Verification items for the finished model (mm, model axes). Coordinates: 2 decimals unless noted, no trailing zeros. Write each loop counter-clockwise with the first axis right and the second up, starting at its lowest first coordinate (ties: lowest second). Pieces come first, ordered by that corner, then holes. Notation, with made-up numbers: (35, -20) -> (78, -20) arc R25 cw to (78, -8) -> close; hole circle Ø10 at (54, 9.25). An arc over 180 degrees is marked (long way). Answer in a Markdown table with one row per item.
```python
from build123d import *

# Parameters (mm, degrees)
F1_DEPTH = 49


with BuildPart() as f1:
    # F0 (on Top) → F1 (new body)
    with BuildSketch(Plane.XY):
        with BuildLine():
            ThreePointArc((-1.772759, -1.023503), (-0.823705, -3.314722), (-0.5, -5.773503))
            Line((-0.5, -5.773503), (0.5, -5.773503))
            ThreePointArc((0.5, -5.773503), (0.823705, -3.314722), (1.772759, -1.023503))
            ThreePointArc((1.772759, -1.023503), (0, -2.047005), (-1.772759, -1.023503))
        make_face()
        with BuildLine():
            Line((-4.75, 3.319764), (-5.25, 2.453739))
            ThreePointArc((-5.25, 2.453739), (-3.282486, 0.944012), (-1.772759, -1.023503))
            ThreePointArc((-1.772759, -1.023503), (-1.772759, 1.023503), (0, 2.047005))
            ThreePointArc((0, 2.047005), (-2.458781, 2.37071), (-4.75, 3.319764))
        make_face()
        with BuildLine():
            ThreePointArc((0, 2.047005), (-1.772759, 1.023503), (-1.772759, -1.023503))
            ThreePointArc((-1.772759, -1.023503), (0, -2.047005), (1.772759, -1.023503))
            ThreePointArc((1.772759, -1.023503), (1.977255, -0.529804), (2.047005, 0))
            ThreePointArc((2.047005, 0), (1.447451, 1.447451), (0, 2.047005))
        make_face()
        with BuildLine():
            ThreePointArc((4.75, 3.319764), (2.458781, 2.37071), (0, 2.047005))
            ThreePointArc((0, 2.047005), (1.447451, 1.447451), (2.047005, 0))
            ThreePointArc((2.047005, 0), (1.977255, -0.529804), (1.772759, -1.023503))
            ThreePointArc((1.772759, -1.023503), (3.282486, 0.944012), (5.25, 2.453739))
            Line((5.25, 2.453739), (4.75, 3.319764))
        make_face()
    extrude(amount=-F1_DEPTH)


solid = f1.part
```
1. Section check A-A, the plane z = -23. Record the boundary of the cut face in (x, y), plus the area to 3 significant figures.
Geometry says:
| item | result |
|---|---|
| outline | (-5.25, 2.45) arc R9.5 cw to (-1.77, -1.02) arc R9.5 cw to (-0.5, -5.77) -> (0.5, -5.77) arc R9.5 cw to (1.77, -1.02) arc R9.5 cw to (5.25, 2.45) -> (4.75, 3.32) arc R9.5 cw to (0, 2.05) arc R9.5 cw to (-4.75, 3.32) -> close |
| area | 31.4 mm^2 |
2. Section check C-C, the plane y = -1.75. Record the boundary of the cut face in (x, z).
Geometry says:
| item | result |
|---|---|
| outline | (-1.39, -49) -> (1.39, -49) -> (1.39, 0) -> (-1.39, 0) -> close |
3. Thickness scan on line 1 (Y direction, x = 0.25, z = -8); line 2 (X direction, y = 3, z = -24.5). Record the ranges inside material, lowest first. Write a range as from..to.
Geometry says:
| item | result |
|---|---|
| line 1 | -5.77..2.05 |
| line 2 | -4.93..-4.15, 4.15..4.93 |
4. Section check B-B, the plane x = 4.25. Record the boundary of the cut face in (y, z), plus the area to 3 significant figures.
Geometry says:
| item | result |
|---|---|
| outline | (1.79, -49) -> (3.05, -49) -> (3.05, 0) -> (1.79, 0) -> close |
| area | 61.8 mm^2 |
5. Depth check by flat-ended pin: P1, Ø1.5, axis at x = 2, y = -1, coming from the +Z side; P2, Ø5, axis at x = -2, z = -6.5, coming from the +Y side; P3, Ø3, axis at y = 0.5, z = -18, coming from the -X side; P4, Ø3, axis at y = -1, z = -38.5, coming from the +X side. Enter the tip coordinate at first touch or a pass-through.
Geometry says:
| item | result |
|---|---|
| P1 | z = 0 |
| P2 | y = 3.18 |
| P3 | x = -4.54 |
| P4 | x = 2.87 |
